Autodesk Inventor part; units mm, degrees
ref_plane "YZ Plane" through (0, 0, 0) normal (1, 0, 0) x (0, 1, 0)
ref_plane "XZ Plane" through (0, 0, 0) normal (0, 1, 0) x (-1, 0, 0)
ref_plane "XY Plane" through (0, 0, 0) normal (0, 0, 1) x (1, 0, 0)
sketch "Sketch1" plane through (0, 0, 0) normal (0, 1, 0) x (-1, 0, 0)
  circle A0 centre (0, 0) radius 127.5
  dimension "d0" = 255
extrude "Extrusion1" add sketch "Sketch1" along normal blind 6
sketch "Sketch2" plane through (0, 6, 0) normal (0, 1, 0) x (1, 0, 0)
  circle A0 centre (0, 0) radius 127.5
  circle A1 centre (0, 0) radius 60
  dimension "d4" = 120
extrude "Extrusion2" add sketch "Sketch2" along normal blind 22 contours A1
sketch "Sketch3" plane through (0, 28, 0) normal (0, 1, 0) x (1, 0, 0)
  circle A0 centre (0, 0) radius 60
  circle A1 centre (0, 30) radius 7.5
  line L0 (0, 30) -> (0, 0) construction
  dimension "d8" = 15
  dimension "d16" = 30
extrude "Extrusion3" cut sketch "Sketch3" against normal through all contours A1
pattern_circular "Circular Pattern1" count 3 over 360 about axis through (0, 6, 0) along (0, 1, 0) of "Extrusion3"
properties part number "rotor"
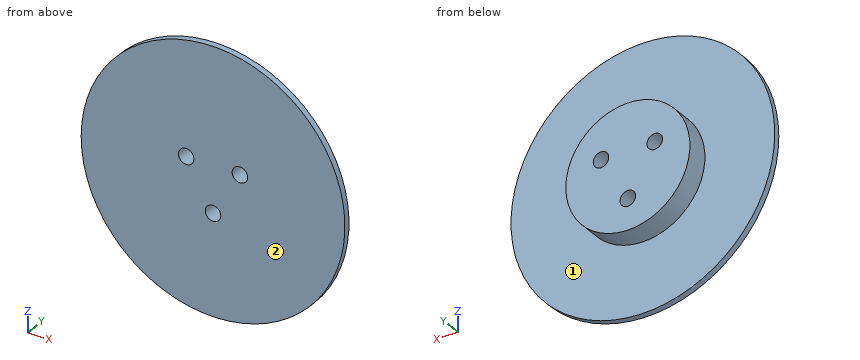
Geometry check sheet. Reference: the model listing, model coordinates, mm. Face numbers are marked on the shaded views. A direction names the side the tool comes from. Coordinates: 2 decimals unless noted, no trailing zeros. Write each loop counter-clockwise with the first axis right and the second up, starting at its lowest first coordinate (ties: lowest second). Pieces come first, ordered by that corner, then holes. Notation, with made-up numbers: (-37.75, 83) -> (-26.75, 83) arc R29 ccw to (-26.75, 121) -> close; hole circle Ø1 at (42.5, -25.75). An arc over 180 degrees is marked (long way). One line per question, with ' | ' between items.
1. Thickness scan on probe 1 along Z at (x, y) = (0, 12.75); probe 2 along X at (y, z) = (18, -2); probe 3 along Y at (x, z) = (-34, -65). Record the ranges inside material, lowest first. Write a range as from..to.
Answers:
probe 1: z = -60..-37.5, -22.5..60 | probe 2: x = -59.97..59.97 | probe 3: y = 0..6
2. Depth check by flat-ended pin: pin 1 Ø8 at (y, z) = (13, 52.5) entering from +X; pin 2 Ø10 at (x, y) = (39.5, 14.5) entering from +Z; pin 3 Ø12 at (x, y) = (52.5, 3.5) entering from -Z; pin 4 Ø8 at (x, z) = (-13.5, -50.5) entering from -Y. Enter the tip coordinate at first touch or a pass-through.
Answers:
pin 1: stops at x = 35.32 | pin 2: stops at z = 49.09 | pin 3: stops at z = -118.72 | pin 4: stops at y = 0
3. Set-up check for the marked faces 1 and 2: record each of +Z, -Z, +X, -X, +Y, -Y from which the full face is reachable in a straight line by a thin tool's end or side.
Answers:
face 1: +Y | face 2: +Z, -Z, +X, -X, -Y
4. Cross-section at D-D on x = 45. Record the cut outline in (y, z).
Answers:
outline: (0, -119.29) -> (6, -119.29) -> (6, -39.69) -> (28, -39.69) -> (28, 39.69) -> (6, 39.69) -> (6, 119.29) -> (0, 119.29) -> close
5. Cross-section at A-A on x = 0. Record the cut outline in (y, z).
Answers:
outline: (0, -127.5) -> (6, -127.5) -> (6, -60) -> (28, -60) -> (28, -37.5) -> (0, -37.5) -> close; (0, -22.5) -> (28, -22.5) -> (28, 60) -> (6, 60) -> (6, 127.5) -> (0, 127.5) -> close
6. Cross-section at B-B on z = 0. Record the cut outline in (x, y), and give its area (3 significant figures).
Answers:
outline: (-127.5, 0) -> (127.5, 0) -> (127.5, 6) -> (60, 6) -> (60, 28) -> (-60, 28) -> (-60, 6) -> (-127.5, 6) -> close | area: 4,170 mm²
7. Cross-section at C-C on z = -30. Record the cut outline in (x, y).
Answers:
outline: (-123.92, 0) -> (-7.5, 0) -> (-7.5, 28) -> (-51.96, 28) -> (-51.96, 6) -> (-123.92, 6) -> close; (7.5, 0) -> (123.92, 0) -> (123.92, 6) -> (51.96, 6) -> (51.96, 28) -> (7.5, 28) -> close
